For this review, take the finished solid that the model builds, in its own axes (mm). A direction names the side the tool comes from. Give positions to 0.01 mm unless a question says otherwise; leave off trailing zeros. Order: outer loops, then holes, each group sorted by start corner. A loop starts at its lowest first (then second) coordinate and runs counter-clockwise, first axis right, second up. Notation, with made-up numbers: (30.25, 5) - (51.25, 5) arc R11 ccw to (51.25, 20) - close; hole circle Ø1 at (52, 26). An arc over 180 degrees is marked (long way). Use a Markdown table: item, result. Add a question column.
1) Machinability: for faces 4 (the face through (-1.08, -4.88, 32.74)), 5 (the face through (8.8, -0.6, 4.9)), 6 (the face through (0, 0, -13)), which of the approach directions +Z, -Z, +X, -X, +Y, -Y give a long, thin tool a straight path to every point of the face, cutting with its end or side? Answer none if there is none.
2) Mouldability with a two-part tool opening along Y and no side actions: class faces 1 (the face through (0.75, 0.03, -8.08)), 2 (the face through (-8, 0, 10)), 3 (the face through (0, 0, 33.5)) as released by +Y, released by -Y, zero draft, split by the parting line, or undercut.
3) We need section C-C on z = 27. Write out the cut boundary in (x, y).
4) We need section D-D on z = -1.5. Write out the cut boundary in (x, y).
5) Wall thickness on L1, parallel to Z at x = 5, y = 9; L2, parallel to Y at x = 8.75, z = 7; L3, parallel to Z at x = -3.5, y = 3.5: over which ranges is each line inside the solid? List them lowest first.
6) Clearance check with flat-ended pins moving along their axes: P1, Ø2.5, axis at x = 8, y = 0, coming from the -Z side; P2, Ø3, axis at x = 9, z = 28.5, coming from the -Y side; P3, Ø5, axis at y = 8, z = 12.5, coming from the -X side. State where each tip first meets the part, or that it passes through.
7) We need section A-A on y = 0. Write out the cut boundary in (x, z).
8) We need section B-B on x = 0. Write out the cut boundary in (y, z), then the cut area to 3 significant figures.
```python
from build123d import *

# Parameters (mm, degrees)
SKETCH1_R           = 14
BOSS_EXTRUDE1_DEPTH = 32
SKETCH2_R           = 5
BOSS_EXTRUDE2_DEPTH = 1.5
BOSS_EXTRUDE3_START = 3.5
SKETCH3_R           = 5
BOSS_EXTRUDE3_DEPTH = 3.5
SKETCH4_R           = 0.75
BOSS_EXTRUDE4_DEPTH = 9.5
SKETCH5_R           = 1
CUT_EXTRUDE1_DEPTH  = 10
FILLET1_R           = 1
FILLET2_R           = 0.2


with BuildPart() as part:
    # Sketch1 → Boss-Extrude1 (new body)
    with BuildSketch(Plane.XY):
        Circle(SKETCH1_R)
    extrude(amount=BOSS_EXTRUDE1_DEPTH)

    # Sketch2 → Boss-Extrude2 (add)
    with BuildSketch(Plane.XY.offset(32)):
        Circle(SKETCH2_R)
    extrude(amount=BOSS_EXTRUDE2_DEPTH)

    # Sketch3 → Boss-Extrude3 (add)
    with BuildSketch(Plane(origin=(0, 0, 0), x_dir=(-1, 0, 0), z_dir=(0, 0, -1)).offset(BOSS_EXTRUDE3_START)):
        with Locations(Location((0, 0, 0), (0, 0, 180))):
            Circle(SKETCH3_R)
    extrude(amount=-BOSS_EXTRUDE3_DEPTH)

    # Sketch4 → Boss-Extrude4 (add)
    with BuildSketch(Plane(origin=(0, 0, -3.5), x_dir=(-1, 0, 0), z_dir=(0, 0, -1))):
        Circle(SKETCH4_R)
    extrude(amount=BOSS_EXTRUDE4_DEPTH)

    # Sketch5 → Cut-Extrude1 (cut)
    with BuildSketch(Plane(origin=(0, 0, 0), x_dir=(-1, 0, 0), z_dir=(0, 0, -1))):
        with Locations((8, 0)):
            Circle(SKETCH5_R)
        with Locations((-8, 0)):
            Circle(SKETCH5_R)
    extrude(amount=-CUT_EXTRUDE1_DEPTH, mode=Mode.SUBTRACT)

    # Fillet1
    fillet1_edges = [part.edges().sort_by_distance(p)[0] for p in [
        (-14, 0, 0),
    ]]
    fillet(fillet1_edges, radius=FILLET1_R)

    # Fillet2
    fillet2_edges = [part.edges().sort_by_distance(p)[0] for p in [
        (0.75, 0, -13),
    ]]
    fillet(fillet2_edges, radius=FILLET2_R)


solid = part.part
```
Checked values:
| question | item | result |
|---|---|---|
| 1 | face 4 | +Z |
| 1 | face 5 | -Z |
| 1 | face 6 | -Z, +X, -X, +Y, -Y |
| 2 | face 1 | split by the parting line |
| 2 | face 2 | undercut |
| 2 | face 3 | zero draft |
| 3 | outline | circle Ø28 at (0, 0) |
| 4 | outline | circle Ø10 at (0, 0) |
| 5 | L1 | 0 to 32 |
| 5 | L2 | -10.93 to -0.66, 0.66 to 10.93 |
| 5 | L3 | -3.5 to 33.5 |
| 6 | P1 | z = 0 |
| 6 | P2 | y = -11.82 |
| 6 | P3 | x = -12.87 |
| 7 | outline | (-14, 1) arc R1 ccw to (-13, 0) - (-9, 0) - (-9, 10) - (-7, 10) - (-7, 0) - (-5, 0) - (-5, -3.5) - (-0.75, -3.5) - (-0.75, -12.8) arc R0.2 ccw to (-0.55, -13) - (0.55, -13) arc R0.2 ccw to (0.75, -12.8) - (0.75, -3.5) - (5, -3.5) - (5, 0) - (7, 0) - (7, 10) - (9, 10) - (9, 0) - (13, 0) arc R1 ccw to (14, 1) - (14, 32) - (5, 32) - (5, 33.5) - (-5, 33.5) - (-5, 32) - (-14, 32) - close |
| 8 | outline | (-14, 1) arc R1 ccw to (-13, 0) - (-5, 0) - (-5, -3.5) - (-0.75, -3.5) - (-0.75, -12.8) arc R0.2 ccw to (-0.55, -13) - (0.55, -13) arc R0.2 ccw to (0.75, -12.8) - (0.75, -3.5) - (5, -3.5) - (5, 0) - (13, 0) arc R1 ccw to (14, 1) - (14, 32) - (5, 32) - (5, 33.5) - (-5, 33.5) - (-5, 32) - (-14, 32) - close |
| 8 | area | 960 mm² |
